from build123d import *

# Parameters (mm, degrees)
BOSS_EXTRUDE1_DEPTH = 40
FILLET2_SIZE        = 15
FILLET2_SIZE_2      = 4
FILLET3_SIZE        = 15
FILLET3_SIZE_2      = 4
FILLET4_SIZE        = 15
FILLET4_SIZE_2      = 4
FILLET5_SIZE        = 4
FILLET5_SIZE_2      = 15
FILLET6_R           = 3
FILLET7_R           = 3
FILLET8_R           = 0.7
FILLET9_R           = 10
FILLET10_R          = 10
SKETCH2_R           = 2.75
CUT_EXTRUDE1_DEPTH  = 178.22584477
FILLET11_R          = 4


with BuildPart() as part:
    # Sketch1 → Boss-Extrude1 (new body)
    with BuildSketch(Plane.XY):
        with BuildLine():
            Line((41.5, 24), (0, 24))
            Line((0, 24), (-48.376623377, -125))
            Line((-48.376623377, -125), (-80, -125))
            Line((-80, -125), (-80, -130))
            Line((-80, -130), (7.792207792, -130))
            Line((7.792207792, -130), (7.792207792, -125))
            Line((7.792207792, -125), (-40.584415584, -125))
            Line((-40.584415584, -125), (0, 0))
            Line((0, 0), (41.5, 0))
            Line((41.5, 0), (41.5, -4))
            Line((41.5, -4), (52.5, -4))
            Line((52.5, -4), (52.5, 4))
            ThreePointArc((52.5, 4), (50.5, 6), (48.5, 4))
            Line((48.5, 4), (48.5, 0))
            Line((48.5, 0), (45.5, 0))
            Line((45.5, 0), (45.5, 4))
            Line((45.5, 4), (4, 4))
            Line((4, 4), (4, 20))
            Line((4, 20), (45.5, 20))
            Line((45.5, 20), (45.5, 24))
            Line((45.5, 24), (48.5, 24))
            Line((48.5, 24), (48.5, 20))
            ThreePointArc((48.5, 20), (50.5, 18), (52.5, 20))
            Line((52.5, 20), (52.5, 28))
            Line((52.5, 28), (41.5, 28))
            Line((41.5, 28), (41.5, 24))
        make_face()
    extrude(amount=BOSS_EXTRUDE1_DEPTH)

    # Fillet2
    # an asymmetric fillet: 15, 4 mm, written as the material it takes off along each edge
    with BuildSketch(Plane(origin=(45.5, 20, -37.5), x_dir=(-1, 0, 0), z_dir=(0, 0, 1))) as fillet2_piece_1:
        with BuildLine():
            Bezier((FILLET2_SIZE, 0), (0, 0), (0, -FILLET2_SIZE_2), weights=[1, 0.707106781, 1])
            Line((0, -FILLET2_SIZE_2), (0, 0))
            Line((0, 0), (FILLET2_SIZE, 0))
        make_face()
    extrude(amount=115, mode=Mode.SUBTRACT)

    # Fillet3
    # an asymmetric fillet: 15, 4 mm, written as the material it takes off along each edge
    with BuildSketch(Plane(origin=(45.5, 4, -37.5), x_dir=(-1, 0, 0), z_dir=(0, 0, 1))) as fillet3_piece_1:
        with BuildLine():
            Bezier((FILLET3_SIZE, 0), (0, 0), (0, FILLET3_SIZE_2), weights=[1, 0.707106781, 1])
            Line((0, FILLET3_SIZE_2), (0, 0))
            Line((0, 0), (FILLET3_SIZE, 0))
        make_face()
    extrude(amount=115, mode=Mode.SUBTRACT)

    # Fillet4
    # an asymmetric fillet: 15, 4 mm, written as the material it adds along each edge
    with BuildSketch(Plane(origin=(41.5, 24, 0), x_dir=(-1, 0, 0), z_dir=(0, 0, 1))) as fillet4_piece_1:
        with BuildLine():
            Bezier((FILLET4_SIZE, 0), (0, 0), (0, -FILLET4_SIZE_2), weights=[1, 0.707106781, 1])
            Line((0, -FILLET4_SIZE_2), (0, 0))
            Line((0, 0), (FILLET4_SIZE, 0))
        make_face()
    extrude(amount=40)

    # Fillet5
    # an asymmetric fillet: 15, 4 mm, written as the material it adds along each edge
    with BuildSketch(Plane(origin=(41.5, 0, 0), x_dir=(0, -1, 0), z_dir=(0, 0, 1))) as fillet5_piece_1:
        with BuildLine():
            Bezier((FILLET5_SIZE, 0), (0, 0), (0, -FILLET5_SIZE_2), weights=[1, 0.707106781, 1])
            Line((0, -FILLET5_SIZE_2), (0, 0))
            Line((0, 0), (FILLET5_SIZE, 0))
        make_face()
    extrude(amount=40)

    # Fillet6
    fillet6_edges = [part.edges().sort_by_distance(p)[0] for p in [
        (4, 4, 20),
        (4, 20, 20),
    ]]
    fillet(fillet6_edges, radius=FILLET6_R)

    # Fillet7
    fillet7_edges = [part.edges().sort_by_distance(p)[0] for p in [
        (52.5, -4, 20),
        (41.5, -4, 20),
        (41.5, 28, 20),
        (52.5, 28, 20),
    ]]
    fillet(fillet7_edges, radius=FILLET7_R)

    # Fillet8
    fillet8_edges = [part.edges().sort_by_distance(p)[0] for p in [
        (45.5, 0, 20),
        (48.5, 0, 20),
        (48.5, 24, 20),
        (45.5, 24, 20),
    ]]
    fillet(fillet8_edges, radius=FILLET8_R)

    # Fillet9
    fillet9_edges = [part.edges().sort_by_distance(p)[0] for p in [
        (0, 0, 20),
        (0, 24, 20),
    ]]
    fillet(fillet9_edges, radius=FILLET9_R)

    # Fillet10
    fillet10_edges = [part.edges().sort_by_distance(p)[0] for p in [
        (-48.376623377, -125, 20),
        (-40.584415584, -125, 20),
    ]]
    fillet(fillet10_edges, radius=FILLET10_R)

    # Sketch2 → Cut-Extrude1 (cut, through all)
    with BuildSketch(Plane(origin=(0, -125, 0), x_dir=(1, 0, 0), z_dir=(0, 1, 0))):
        with Locations(Location((-67.82186874, -20, 0), (0, 0, 270))):
            Circle(SKETCH2_R)
        with Locations(Location((-9.515793598, -20, 0), (0, 0, 270))):
            Circle(SKETCH2_R)
    extrude(amount=-CUT_EXTRUDE1_DEPTH, mode=Mode.SUBTRACT)

    # Fillet11
    fillet11_edges = [part.edges().sort_by_distance(p)[0] for p in [
        (7.792207792, -125, 20),
        (-80, -125, 20),
    ]]
    fillet(fillet11_edges, radius=FILLET11_R)


solid = part.part
Here's how the part is built. I have some questions about the finished solid (model axes, mm). A direction names the side the tool comes from. Give positions to 0.01 mm unless a question says otherwise; leave off trailing zeros. Order: outer loops, then holes, each group sorted by start corner. A loop starts at its lowest first (then second) coordinate and runs counter-clockwise, first axis right, second up. Notation, with made-up numbers: M 13,-5 L 23,-5 A13 ccw 23,13 Z; hole C 39.5,62 d1. An arc over 180 degrees is marked long. Answer as a JSON object with one key per item and string values. Group by question number.
1) Suppose I cut it at C-C, the plane x = -62.5. Write out the boundary of the cut face in (y, z).
2) Suppose I cut it at B-B, the plane x = -34. Write out the boundary of the cut face in (y, z).
3) Please list where these lines run through material, in increasing order: L1, parallel to X at y = -128.5, z = 20; L2, parallel to Y at x = 9, z = 7; L3, parallel to X at y = -127, z = 20. Write a range as [from, to].
4) Suppose I cut it at D-D, the plane y = -76. Write out the boundary of the cut face in (x, z), plus the area to 3 significant figures.
5) I'm going to push flat-ended pins straight in: pin 1 Ø16.5 at (x, z) = (-69, 29.5) entering from +Y; pin 2 Ø3.5 at (y, z) = (2.5, 21) entering from -X; pin 3 Ø10 at (y, z) = (-108.5, 26) entering from +X; pin 4 Ø5 at (x, y) = (-16, -64) entering from -Z. Where does each tip first touch, or does it pass through?
6) Suppose I cut it at A-A, the plane z = 20. Count the separate pieces of the cut face and the enclosed holes in it, plus the area to 3 significant figures.
7) We'd pull the mould along Y, two halves only. Please class faces 1 (the flat face through (-63, -125, 20)), 2 (the flat face through (52.5, 22, 20)), 3 (the flat face through (4, 12, 20)): pulls with the +Y half, pulls with the -Y half, needs draft (parallel to the pull), parting line crosses it, or undercut.
8) On a 3-axis mill with a long thin cutter (end or side, diameter ignored), from which of +Z, -Z, +X, -X, +Y, -Y can I reach the whole of each face in a straight line? I mean faces 4 (the cylindrical face through (6.65, -126.2, 20.28)), 5 (the cylindrical face through (50.5, 6, 19.7)), 6 (the flat face through (52.5, 1, 20)), 7 (the flat face through (46, -4, 20)), 8 (the flat face through (-23.88, -49.55, 19.72)). Say none if no direction works.
Results found:
{
 "1": {"outline": "M -130,0 L -125,0 L -125,40 L -130,40 Z"},
 "2": {"outline": "M -130,0 L -121.96,0 L -121.96,40 L -130,40 Z; M -104.72,0 L -80.72,0 L -80.72,40 L -104.72,40 Z"},
 "3": {"L1": "[-79.97, -70.57], [-65.07, -12.27], [-6.77, 7.76]", "L2": "[0, 4], [20, 24]", "L3": "[-79.46, -70.57], [-65.07, -12.27], [-6.77, 7.26]"},
 "4": {"outline": "M -32.47,0 L -24.68,0 L -24.68,40 L -32.47,40 Z", "area": "312 mm²"},
 "5": {"pin 1": "y = -125", "pin 2": "x = -7.55", "pin 3": "x = -33.6", "pin 4": "through"},
 "6": {"separate pieces": "3", "enclosed holes": "0", "area": "2,060 mm²"},
 "7": {"face 1": "pulls with the +Y half", "face 2": "needs draft", "face 3": "undercut"},
 "8": {"face 4": "+Z, -Z, +X", "face 5": "+Z, -Z", "face 6": "+Z, -Z, +X, +Y, -Y", "face 7": "+Z, -Z, +X, -Y", "face 8": "+Z, -Z, -X, +Y"}
}
